Job drawing, mm, ordinate dimensions from the low corner. One solid piece. A direction names the side the tool comes from. Round coordinates to 2 decimals unless told otherwise and drop trailing zeros. Loops run counter-clockwise (first coordinate to the right, second up) from the corner with the lowest first, then second, coordinate; pieces in that order, holes last.
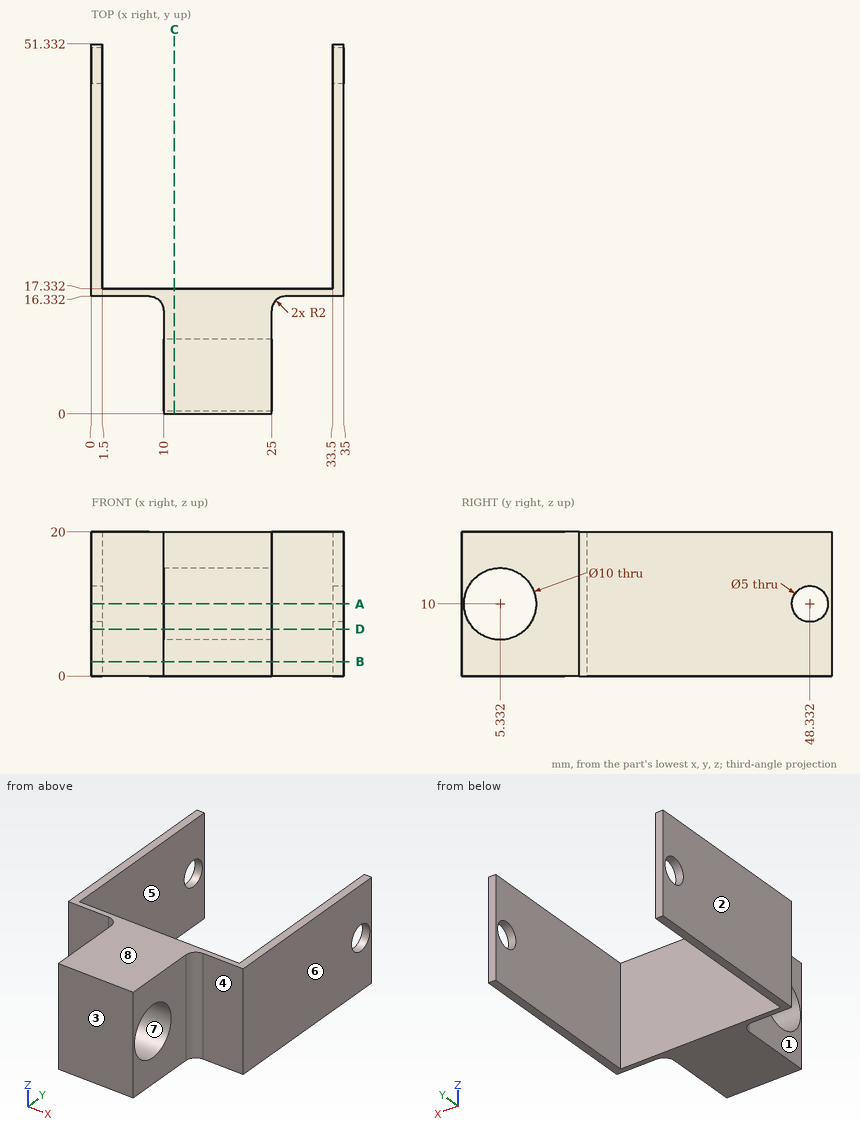
1) Drop flat-ended pins along their axis: pin 1 Ø6.5 at (y, z) = (48.33, 10) entering from +X; pin 2 Ø6.5 at (x, z) = (2.5, 12.5) entering from -Y; pin 3 Ø11.5 at (y, z) = (5.33, 10) entering from +X; pin 4 Ø3 at (x, z) = (17, 15) entering from +Y. Give the stop position or say it passes through.
Values:
pin 1: stops at x = 35
pin 2: stops at y = 16.33
pin 3: stops at x = 25
pin 4: stops at y = 17.33
2) Tool access for the marked faces 1, 2, 3, 4 and 5: list every direction of +Z, -Z, +X, -X, +Y, -Y with a clear straight run to the whole face (end or side of a thin tool).
Values:
face 1: +Z, -Z, -X, -Y
face 2: +Z, -Z, -X, +Y, -Y
face 3: +Z, -Z, +X, -X, -Y
face 4: +Z, -Z, +X, -Y
face 5: +Z, -Z, +Y
3) Wall check: line 1 along X through (y, z) = (37.5, 7.75); line 2 along Y through (x, z) = (34.2, 10); line 3 along Y through (x, z) = (5, 3.75). Give the ranges that are in metal, low to high.
Values:
line 1: x = 0 to 1.5, 33.5 to 35
line 2: y = 16.33 to 45.83, 50.83 to 51.33
line 3: y = 16.33 to 17.33
4) Slice it at C-C, the plane x = 11.5. Give the cut face in (y, z).
Values:
outline: (0, 0) - (17.33, 0) - (17.33, 20) - (0, 20) - close; hole circle Ø10 at (5.33, 10)
5) Slice it at D-D, the plane z = 6.5. Give the cut face in (x, y).
Values:
outline: (0, 16.33) - (8, 16.33) arc R2 cw to (10, 14.33) - (10, 8.9) - (25, 8.9) - (25, 14.33) arc R2 cw to (27, 16.33) - (35, 16.33) - (35, 51.33) - (33.5, 51.33) - (33.5, 17.33) - (1.5, 17.33) - (1.5, 51.33) - (0, 51.33) - close; (10, 0) - (25, 0) - (25, 1.76) - (10, 1.76) - close
6) Slice it at A-A, the plane z = 10. Give the cut face in (x, y).
Values:
outline: (0, 16.33) - (8, 16.33) arc R2 cw to (10, 14.33) - (10, 10.33) - (25, 10.33) - (25, 14.33) arc R2 cw to (27, 16.33) - (35, 16.33) - (35, 45.83) - (33.5, 45.83) - (33.5, 17.33) - (1.5, 17.33) - (1.5, 45.83) - (0, 45.83) - close; (0, 50.83) - (1.5, 50.83) - (1.5, 51.33) - (0, 51.33) - close; (10, 0) - (25, 0) - (25, 0.33) - (10, 0.33) - close; (33.5, 50.83) - (35, 50.83) - (35, 51.33) - (33.5, 51.33) - close
7) Mould opens along Z. For the marked faces 6, 7 and 8 say: released by +Z, released by -Z, zero draft, split by the parting line, or undercut.
Values:
face 6: zero draft
face 7: undercut
face 8: released by +Z
8) Slice it at B-B, the plane z = 2. Give the cut face in (x, y), then the cut area to 3 significant figures.
Values:
outline: (0, 16.33) - (8, 16.33) arc R2 cw to (10, 14.33) - (10, 0) - (25, 0) - (25, 14.33) arc R2 cw to (27, 16.33) - (35, 16.33) - (35, 51.33) - (33.5, 51.33) - (33.5, 17.33) - (1.5, 17.33) - (1.5, 51.33) - (0, 51.33) - close
area: 384 mm2
